from build123d import *

# Parameters (mm, degrees)
F2_DEPTH = 10
F5_DEPTH = 1.5875


with BuildPart() as f2:
    # F1 (on Right) → F2 (new body)
    with BuildSketch(Plane.YZ):
        Polygon((-10.5, 14.2), (-10.5, 15.2), (-7.96, 15.2), (-7.96, 16.7875), (-13.7, 16.7875), (-13.7, 12.6125), (-7.96, 12.6125), (-7.96, 14.2), align=None)
        Polygon((-24.2, -0.5), (-24.2, 0.5), (-21.66, 0.5), (-21.66, 2.0875), (-27.4, 2.0875), (-27.4, -2.0875), (-21.66, -2.0875), (-21.66, -0.5), align=None)
        Polygon((-5.74, 0.5), (-3.2, 0.5), (-3.2, -0.5), (-5.74, -0.5), (-5.74, -2.0875), (0, -2.0875), (0, 2.0875), (-5.74, 2.0875), align=None)
    extrude(amount=F2_DEPTH)



with BuildPart() as f3_1:
    # F3: instance of F2
    add(f2.part.mirror(Plane.XZ))


with BuildPart() as f2_1:
    add(f2.part)

    add(f3_1.part)  # F5 merges F3_1
    # F4 (on face) → F5 (join)
    with BuildSketch(Plane(origin=(0, 0, 0), x_dir=(0, -1, 0), z_dir=(-1, 0, 0))):
        Polygon((13.7, 16.7875), (-13.7, 16.7875), (-13.7, 2.0875), (-27.4, 2.0875), (-27.4, -2.0875), (27.4, -2.0875), (27.4, 2.0875), (13.7, 2.0875), align=None)
    extrude(amount=F5_DEPTH)


solid = f2_1.part
For this review, take the finished solid that the model builds, in its own axes (mm). A direction names the side the tool comes from. Round coordinates to 2 decimals unless told otherwise and drop trailing zeros. Write each loop counter-clockwise with the first axis right and the second up, starting at its lowest first coordinate (ties: lowest second). Pieces come first, ordered by that corner, then holes. Notation, with made-up numbers: (61.25, 6) - (71.25, 6) arc R26 ccw to (71.25, 20) - close; hole circle Ø1 at (44, -34.5). An arc over 180 degrees is marked (long way). Use a Markdown table: item, result.
Q1. We need section C-C (z = 7). Give the boundary of the cut face in (x, y), plus the area to 3 significant figures.
Derived:
| item | result |
|---|---|
| outline | (-1.59, -13.7) - (0, -13.7) - (0, 13.7) - (-1.59, 13.7) - close |
| area | 43.5 mm2 |
Q2. The part is to be moulded in two halves that separate along Y. For faces 1 (the flat face through (3, -13.7, 13)), 2 (the flat face through (4, -24, 2.088)), 3 (the flat face through (5, -4, -0.5)), say which applies: pulls with the +Y half, pulls with the -Y half, needs draft (parallel to the pull), parting line crosses it, or undercut.
Derived:
| item | result |
|---|---|
| face 1 | pulls with the -Y half |
| face 2 | needs draft |
| face 3 | undercut |
Q3. We need section B-B (x = 1.75). State how many separate pieces and enclosed holes the cut face has, plus the area to 3 significant figures.
Derived:
| item | result |
|---|---|
| separate pieces | 5 |
| enclosed holes | 0 |
| area | 129 mm2 |
Q4. Clearance check with flat-ended pins moving along their axes: pin 1 (1.3 mm diameter, centred on x = 3.5, y = -23, fed in from +Z); pin 2 (0.8 mm diameter, centred on x = 5, z = 13.5, fed in from +Y); pin 3 (6 mm diameter, centred on x = 2.5, z = 8, fed in from -Y); pin 4 (4 mm diameter, centred on y = -10, z = 12, fed in from +X). State where each tip first meets the part, or that it passes through.
Derived:
| item | result |
|---|---|
| pin 1 | stops at z = 2.09 |
| pin 2 | stops at y = 13.7 |
| pin 3 | stops at y = -13.7 |
| pin 4 | stops at x = 10 |
Q5. We need section A-A (y = -4.5). Give the boundary of the cut face in (x, z).
Derived:
| item | result |
|---|---|
| outline | (-1.59, -2.09) - (10, -2.09) - (10, -0.5) - (0, -0.5) - (0, 0.5) - (10, 0.5) - (10, 2.09) - (0, 2.09) - (0, 16.79) - (-1.59, 16.79) - close |
Q6. Wall thickness on line 1 along Y through (x, z) = (6.5, -0.25); line 2 along Y through (x, z) = (8.5, 14); line 3 along X through (y, z) = (-21.5, -1): over which ranges is each line inside the solid? List them lowest first.
Derived:
| item | result |
|---|---|
| line 1 | y = -27.4 to -24.2, -3.2 to 3.2, 24.2 to 27.4 |
| line 2 | y = -13.7 to -7.96, 7.96 to 13.7 |
| line 3 | x = -1.59 to 0 |
Q7. We need section D-D (y = -17.5). Give the boundary of the cut face in (x, z), plus the area to 3 significant figures.
Derived:
| item | result |
|---|---|
| outline | (-1.59, -2.09) - (0, -2.09) - (0, 2.09) - (-1.59, 2.09) - close |
| area | 6.63 mm2 |
Q8. Machinability: for faces 4 (the flat face through (10, -25, 0)), 5 (the flat face through (5, -10.5, 15)), 6 (the flat face through (4, 23, 2.088)), 7 (the flat face through (-1, 0, 16.788)), 8 (the flat face through (5, -5.74, 1)), which of the approach directions +Z, -Z, +X, -X, +Y, -Y give a long, thin tool a straight path to every point of the face, cutting with its end or side? Answer none if there is none.
Derived:
| item | result |
|---|---|
| face 4 | +Z, -Z, +X, +Y, -Y |
| face 5 | +X |
| face 6 | +Z, +X, -X, +Y |
| face 7 | +Z, +X, -X, +Y, -Y |
| face 8 | +Z, -Z, +X |
